from build123d import *

# Parameters (mm, degrees)
SKETCH1_R             = 27.5
BOSS_EXTRUDE1_DEPTH   = 8
SKETCH2_R             = 7.5
CUT_EXTRUDE1_DEPTH    = 40.705163392
SKETCH3_R             = 1.973316749
CUT_EXTRUDE2_DEPTH    = 6.642946
CIRPATTERN1_START     = 1.357053983
CIRPATTERN1_OUTLINE_R = 1.973316749
CIRPATTERN1_DEPTH     = 6.642946017


# Read off the part's stored shape, not the designer's step: CirPattern1
with BuildPart() as part:
    # Sketch1 → Boss-Extrude1 (new body)
    with BuildSketch(Plane(origin=(0, 0, 0), x_dir=(1, 0, 0), z_dir=(0, 1, 0))):
        with Locations(Location((0, 0, 0), (0, 0, 270))):
            Circle(SKETCH1_R)
    extrude(amount=BOSS_EXTRUDE1_DEPTH)

    # Sketch2 → Cut-Extrude1 (cut, through all)
    with BuildSketch(Plane(origin=(0, 0, 0), x_dir=(1, 0, 0), z_dir=(0, 1, 0))):
        with Locations(Location((0, 0, 0), (0, 0, 270))):
            Circle(SKETCH2_R)
    extrude(amount=CUT_EXTRUDE1_DEPTH, mode=Mode.SUBTRACT)

    # Sketch3 → Cut-Extrude2 (cut)
    with BuildSketch(Plane(origin=(0, 8, 0), x_dir=(1, 0, 0), z_dir=(0, 1, 0))):
        with Locations(Location((-11.709849239, 0, 0), (0, 0, 270))):
            Circle(SKETCH3_R)
    extrude(amount=-CUT_EXTRUDE2_DEPTH, mode=Mode.SUBTRACT)

    # CirPattern1 outline → CirPattern1 (cut)
    with BuildSketch(Plane(origin=(0, 0, 0), x_dir=(1, 0, 0), z_dir=(0, 1, 0)).offset(CIRPATTERN1_START)):
        with Locations((5.85492462, 10.141026915)):
            Circle(CIRPATTERN1_OUTLINE_R)
        with Locations((5.85492462, -10.141026915)):
            Circle(CIRPATTERN1_OUTLINE_R)
    extrude(amount=CIRPATTERN1_DEPTH, mode=Mode.SUBTRACT)


solid = part.part
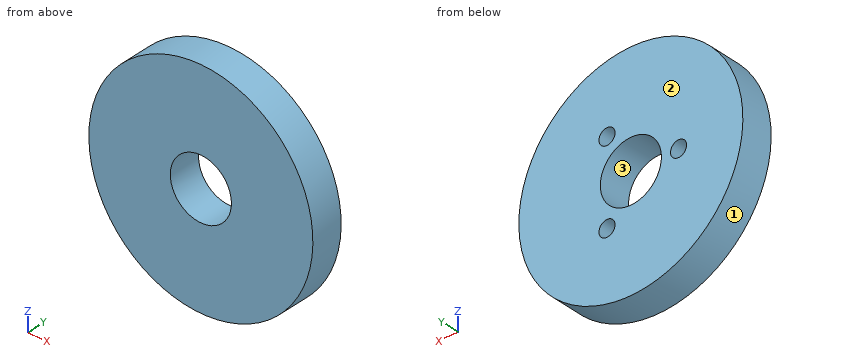
Model file for the job. Use its own axes, mm. Face numbers are marked on the shaded views. Round coordinates to 2 decimals unless told otherwise and drop trailing zeros. Order: outer loops, then holes, each group sorted by start corner. A loop starts at its lowest first (then second) coordinate and runs counter-clockwise, first axis right, second up.
(1) Band-saw the part on A-A (x = 0). List the corners of the cut face in (y, z).
(2) Drill centre lines: line 1 (X direction, y = 2.5, z = 0); line 2 (Z direction, x = -5.5, y = 5.75); line 3 (X direction, y = 7, z = -6). Where is each one in solid material? Low to high.
(3) Band-saw the part on B-B (z = 0). List the corners of the cut face in (x, y), then the cut area to 3 significant figures.
(4) Pin check, flat tips, straight feed: pin 1 (1.2 mm diameter, centred on x = -12.5, z = 0.5, fed in from +Y); pin 2 (3 mm diameter, centred on y = 4.5, z = 6.5, fed in from +X); pin 3 (1 mm diameter, centred on x = -14.5, y = 5, fed in from +Z). Stop position of each tip, or through.
(5) Band-saw the part on C-C (y = 7.25). List the corners of the cut face in (x, z).
(6) Pull direction Z, two halves, no side cores. Call the marked faces 1, 2 and 3: released by +Z, released by -Z, zero draft, split by the parting line, or undercut.
(7) Band-saw the part on D-D (x = -11). List the corners of the cut face in (y, z).
Verdict:
1. outline: (0, -27.5) - (8, -27.5) - (8, -7.5) - (0, -7.5) - close; (0, 7.5) - (8, 7.5) - (8, 27.5) - (0, 27.5) - close
2. line 1: x = -27.5 to -13.68, -9.74 to -7.5, 7.5 to 27.5
2. line 2: z = -26.94 to -5.1, 5.1 to 26.94
2. line 3: x = -26.84 to -4.5, 4.5 to 26.84
3. outline: (-27.5, 0) - (-7.5, 0) - (-7.5, 8) - (-9.74, 8) - (-9.74, 1.36) - (-13.68, 1.36) - (-13.68, 8) - (-27.5, 8) - close; (7.5, 0) - (27.5, 0) - (27.5, 8) - (7.5, 8) - close
3. area: 294 mm2
4. pin 1: stops at y = 1.36
4. pin 2: stops at x = 27.04
4. pin 3: stops at z = 23.67
5. outline: circle Ø55 at (0, 0); hole circle Ø3.95 at (-11.71, 0); hole circle Ø15 at (0, 0); hole circle Ø3.95 at (5.85, -10.14); hole circle Ø3.95 at (5.85, 10.14)
6. face 1: split by the parting line
6. face 2: zero draft
6. face 3: undercut
7. outline: (0, -25.2) - (8, -25.2) - (8, -1.84) - (1.36, -1.84) - (1.36, 1.84) - (8, 1.84) - (8, 25.2) - (0, 25.2) - close
